from build123d import *

# Parameters (mm, degrees)
SKETCH1_R           = 2.25
BOSS_EXTRUDE1_DEPTH = 2.5
SKETCH2_R           = 1.25
BOSS_EXTRUDE2_DEPTH = 12
CHAMFER1_SIZE       = 0.3
CUT_EXTRUDE1_DEPTH  = 2


with BuildPart() as part:
    # Sketch1 → Boss-Extrude1 (new body)
    with BuildSketch(Plane.XY):
        Circle(SKETCH1_R)
    extrude(amount=BOSS_EXTRUDE1_DEPTH)

    # Sketch2 → Boss-Extrude2 (add)
    with BuildSketch(Plane(origin=(0, 0, 0), x_dir=(-1, 0, 0), z_dir=(0, 0, -1))):
        Circle(SKETCH2_R)
    extrude(amount=BOSS_EXTRUDE2_DEPTH)

    # Chamfer1
    chamfer1_edges = [part.edges().sort_by_distance(p)[0] for p in [
        (1.25, 0, -12),
    ]]
    chamfer(chamfer1_edges, length=CHAMFER1_SIZE)

    # Sketch3 → Cut-Extrude1 (cut)
    with BuildSketch(Plane.XY.offset(2.5)):
        Polygon((0, 1.154700538), (-1, 0.577350269), (-1, -0.577350269), (0, -1.154700538), (1, -0.577350269), (1, 0.577350269), align=None)
    extrude(amount=-CUT_EXTRUDE1_DEPTH, mode=Mode.SUBTRACT)


solid = part.part
The listing builds one solid part. Answer for the finished solid, in the listing's coordinates (mm). A direction names the side the tool comes from. Coordinates: 2 decimals unless noted, no trailing zeros. Write each loop counter-clockwise with the first axis right and the second up, starting at its lowest first coordinate (ties: lowest second). Pieces come first, ordered by that corner, then holes. Notation, with made-up numbers: (74, -37) - (119, -37) arc R26 ccw to (119, 0) - close; hole circle Ø7 at (69, 36). An arc over 180 degrees is marked (long way). Return JSON: item names as keys, results as strings.
1. Which of the six approach directions +Z, -Z, +X, -X, +Y, -Y give full straight-line access (tool end or side, diameter ignored) to faces 4 (the face through (1, -1, 0)), 5 (the face through (1, 0, 2)), 6 (the face through (-0.29, 2.23, 1.23))?
Final values:
{"face 4": "-Z", "face 5": "+Z", "face 6": "+Z, -Z"}
2. The part is cut by section C-C on x = -1.9. Determine the outline of the cut face in (y, z).
Final values:
{"outline": "(-1.21, 0) - (1.21, 0) - (1.21, 2.5) - (-1.21, 2.5) - close"}
3. For a pull along X with two mould halves and no side action, classify faces 1 (the face through (0, 0, -12)), 2 (the face through (0.27, -1.22, -5.77)), 3 (the face through (0, 0, 0.5)) as +X half, -X half, draft (parallel to the pull), parting line (faces both ways), or undercut.
Final values:
{"face 1": "draft", "face 2": "parting line", "face 3": "undercut"}
4. Consider line 1 along Z through (x, y) = (-1.25, -0.8); line 2 along X through (y, z) = (0.75, -3); line 3 along X through (y, z) = (0.65, 1.75). Determine where each line is inside the solid, lowest interval first.
Final values:
{"line 1": "0 to 2.5", "line 2": "-1 to 1", "line 3": "-2.15 to -0.87, 0.87 to 2.15"}
5. The part is cut by section B-B on z = -8.75. Determine the outline of the cut face in (x, y), then the cut area to 3 significant figures.
Final values:
{"outline": "circle Ø2.5 at (0, 0)", "area": "4.91 mm^2"}
6. This flat-tipped pin is pushed along its axis until it touches: pin 1 Ø1.6 at (x, y) = (0, 0) entering from +Z. Where does it stop, or does it pass through?
Final values:
{"pin 1": "z = 0.5"}
7. The part is cut by section A-A on y = 0. Determine the outline of the cut face in (x, z).
Final values:
{"outline": "(-2.25, 0) - (-1.25, 0) - (-1.25, -11.7) - (-0.95, -12) - (0.95, -12) - (1.25, -11.7) - (1.25, 0) - (2.25, 0) - (2.25, 2.5) - (1, 2.5) - (1, 0.5) - (-1, 0.5) - (-1, 2.5) - (-2.25, 2.5) - close"}
